from build123d import *

# Parameters (mm, degrees)
SKETCH1_R           = 7
BOSS_EXTRUDE1_DEPTH = 10
BOSS_EXTRUDE2_DEPTH = 12
BOSS_EXTRUDE3_DEPTH = 4
BOSS_EXTRUDE4_START = -15
BOSS_EXTRUDE4_DEPTH = 4


with BuildPart() as part:
    # Sketch1 → Boss-Extrude1 (new body)
    with BuildSketch(Plane(origin=(0, 0, 0), x_dir=(0, 0, -1), z_dir=(1, 0, 0))):
        with BuildLine():
            Line((-45, 35), (45, 35))
            ThreePointArc((45, 35), (52.071067812, 32.071067812), (55, 25))
            Line((55, 25), (55, -35))
            Line((55, -35), (-55, -35))
            Line((-55, -35), (-55, 25))
            ThreePointArc((-55, 25), (-52.071067812, 32.071067812), (-45, 35))
        make_face()
        with Locations((-35, 15)):
            Circle(SKETCH1_R, mode=Mode.SUBTRACT)
        with Locations(Location((35, 15, 0), (0, 0, 180))):
            Circle(SKETCH1_R, mode=Mode.SUBTRACT)
    extrude(amount=BOSS_EXTRUDE1_DEPTH)



with BuildPart() as body_2:
    # Sketch4 → Boss-Extrude2 (new body)
    with BuildSketch(Plane.ZY.offset(-105)):
        Polygon((6, -35), (6, -23), (15, -23), (15, -11), (-15, -11), (-15, -23), (-6, -23), (-6, -35), align=None)
    extrude(amount=BOSS_EXTRUDE2_DEPTH)


with BuildPart() as part_1:
    add(part.part)

    add(body_2.part)  # Boss-Extrude3 merges body 2
    # Sketch5 → Boss-Extrude3 (add, symmetric)
    with BuildSketch(Plane.XY):
        with BuildLine():
            Line((44.783977599, -4.658455723), (93, -11))
            Line((93, -11), (93, -15))
            Line((93, -15), (10, -15))
            Line((10, -15), (10, 35))
            ThreePointArc((10, 35), (19.928078744, 8.624262058), (44.783977599, -4.658455723))
        make_face()
    extrude(amount=BOSS_EXTRUDE3_DEPTH, both=True)

    # Sketch6 → Boss-Extrude4 (add, symmetric)
    with BuildSketch(Plane(origin=(0, 0, 0), x_dir=(1, 0, 0), z_dir=(0, 1, 0)).offset(BOSS_EXTRUDE4_START)):
        Polygon((93, -15), (93, -4), (93, 4), (93, 15), (10, 43), (10, -43), align=None)
    extrude(amount=BOSS_EXTRUDE4_DEPTH, both=True)


solid = part_1.part
Read the model definition and answer for the solid it produces. Units are mm, in the model's axes. A direction names the side the tool comes from. Give positions to 0.01 mm unless a question says otherwise; leave off trailing zeros. Write each loop counter-clockwise with the first axis right and the second up, starting at its lowest first coordinate (ties: lowest second). Pieces come first, ordered by that corner, then holes. Notation, with made-up numbers: (8.5, -10.5) - (33.5, -10.5) arc R15 cw to (33.5, -2.5) - close; hole circle Ø2 at (-36.75, -28.5). An arc over 180 degrees is marked (long way). Use CSV: the item, a comma, the result in double quotes. Start each with the question number.
(1) Find section C-C (y = -17). Give the vertices of the cut face in (x, z), plus the area to 3 significant figures.
(2) Consider line 1 along Y through (x, z) = (7, 35); line 2 along X through (y, z) = (-7.5, -8.5); line 3 along Y through (x, z) = (10.5, -27.5). Determine where each line is inside the solid, lowest interval first.
(3) For faces 1 (the flat face through (99, -17, -15)), 2 (the flat face through (99, -17, 15)), 3 (the flat face through (99, -23, 10)), 4 (the flat face through (30, -3, -4)), determine the directions among +Z, -Z, +X, -X, +Y, -Y from which every point of the face is accessible in a straight line to the end or side of a thin tool.
(4) Find section A-A (y = 15). Give the vertices of the cut face in (x, z), plus the area to 3 significant figures.
(5) Determine the mould class of faces 5 (the flat face through (0, 0, -1)), 6 (the flat face through (42, -19, -1)), 7 (the flat face through (93, -25, 0)), 8 (the flat face through (5, 35, 1)) for opening direction X: +X half, -X half, draft (parallel to the pull), parting line (faces both ways), or undercut.
(6) Find section D-D (x = 40). Give the vertices of the cut face in (y, z), plus the area to 3 significant figures.
(7) Given P1, Ø3.5, axis at x = 99, y = -18, coming from the +Z side; P2, Ø2.5, axis at x = 99.5, z = -11, coming from the -Y side; P3, Ø3, axis at x = 31, z = 3, coming from the +Y side, each flat-ended and moving along its own axis, determine where each tip first touches the part or whether it passes through.
(8) Find section B-B (z = -35). Give the vertices of the cut face in (x, y), plus the area to 3 significant figures.
Findings below:
1,outline,"(0, -55) - (10, -55) - (10, -43) - (93, -15) - (105, -15) - (105, 15) - (93, 15) - (10, 43) - (10, 55) - (0, 55) - close"
1,area,"6,270 mm2"
2,line 1,"-35 to 8, 22 to 35"
2,line 2,"0 to 10"
2,line 3,"-19 to -11"
3,face 1,"-Z, +X, +Y, -Y"
3,face 2,"+Z, +X, +Y, -Y"
3,face 3,"+Z, +X, -Y"
3,face 4,"-Z, +X, +Y"
4,outline,"(0, -55) - (10, -55) - (10, -42) - (0, -42) - close; (0, -28) - (10, -28) - (10, -4) - (15.36, -4) - (15.36, 4) - (10, 4) - (10, 28) - (0, 28) - close; (0, 42) - (10, 42) - (10, 55) - (0, 55) - close"
4,area,"863 mm2"
5,face 5,"-X half"
5,face 6,"undercut"
5,face 7,"undercut"
5,face 8,"draft"
6,outline,"(-19, -32.88) - (-11, -32.88) - (-11, -4) - (-3.73, -4) - (-3.73, 4) - (-11, 4) - (-11, 32.88) - (-19, 32.88) - close"
6,area,"584 mm2"
7,P1,"z = 15"
7,P2,"y = -23"
7,P3,"y = 0.65"
8,outline,"(0, -35) - (10, -35) - (10, -19) - (33.71, -19) - (33.71, -11) - (10, -11) - (10, 8) - (0, 8) - close; (0, 22) - (10, 22) - (10, 35) - (0, 35) - close"
8,area,"750 mm2"
